Autodesk Inventor part; units mm, degrees
ref_plane "YZ Plane" through (0, 0, 0) normal (1, 0, 0) x (0, 1, 0)
ref_plane "XZ Plane" through (0, 0, 0) normal (0, 1, 0) x (-1, 0, 0)
ref_plane "XY Plane" through (0, 0, 0) normal (0, 0, 1) x (1, 0, 0)
sketch "Skizze1" plane through (0, 0, 0) normal (0, 0, 1) x (1, 0, 0)
  line L0 (-58, -45) -> (58, -45)
  line L1 (58, -45) -> (58, 45)
  line L2 (58, 45) -> (-58, 45)
  line L3 (-58, 45) -> (-58, -45)
  line L4 (-58, -45) -> (58, 45) construction
  line L5 (58, -45) -> (-58, 45) construction
  point P0 (0, 0)
  dimension "d0" = 116
  dimension "d1" = 90
extrude "Extrusion1" add sketch "Skizze1" along normal blind 15
sketch "Skizze2" plane through (0, 0, 15) normal (0, 0, 1) x (1, 0, 0)
  line L0 (58, -45) -> (58, 45)
  point P0 (0, 0)
  point P1 (47, 0)
  point P2 (58, 0)
  dimension "d11" = 11
hole "Bohrung1" at (47, 0, 15) direction (0, 0, -1) diameter 4.134 depth 13 tip angle 118
sketch "Skizze4" plane through (0, 0, 15) normal (0, 0, 1) x (1, 0, 0)
  line L0 (-58, -45) -> (58, -45)
  line L1 (58, -45) -> (58, 45)
  point P0 (0, 0)
  point P1 (-35.5, 16)
  point P2 (36, -10)
  dimension "d20" = 35
  dimension "d21" = 61
  dimension "d22" = 22
  dimension "d23" = 71.5
hole "Bohrung3" at (-35.5, 16, 15) at (36, -10, 15) direction (0, 0, -1) diameter 5.5 end through all counterbore diameter 10 counterbore depth 6.5
sketch "Skizze5" plane through (0, 0, 15) normal (0, 0, 1) x (1, 0, 0)
  line L0 (-58, 45) -> (-58, -45)
  circle A0 centre (47, 0) radius 2.067
  point P0 (0, 0)
  point P1 (-46.5721, 0)
  point P2 (-58, 0)
  dimension "d38" = 93.5721
hole "Bohrung4" at (-46.5721, 0, 15) direction (0, 0, -1) diameter 4.134 depth 13 tip angle 118
sketch "Skizze6" plane through (0, 0, 15) normal (0, 0, 1) x (1, 0, 0)
  circle A0 centre (-35.5, 16) radius 2.75
  point P0 (0, 0)
  point P1 (-35.5, -14)
  dimension "d39" = 30
hole "Bohrung5" at (-35.5, -14, 15) direction (0, 0, -1) diameter 5.5 depth 15 counterbore diameter 10 counterbore depth 6.5
sketch "Skizze7" plane through (0, 0, 15) normal (0, 0, 1) x (1, 0, 0)
  point P0 (0, 0)
  point P1 (-46.0168, 35.3976)
hole "Bohrung6" at (-46.0168, 35.3976, 15) direction (0, 0, -1) diameter 3 depth 8 tip angle 118
sketch "Skizze8" plane through (0, 0, 0) normal (0, 0, -1) x (-1, 0, 0)
  line L0 (58, -45) -> (-58, -45)
  line L1 (58, 45) -> (58, -45)
  point P0 (0, 0)
  point P1 (42.6552, 35)
  point P2 (24.6552, -15)
  point P3 (58, 0)
  dimension "d61" = 50
  dimension "d62" = 30
  dimension "d63" = 18
hole "Bohrung7" at (-42.6552, 35, 0) at (-24.6552, -15, 0) direction (0, 0, 1) diameter 4 depth 8 tip angle 118
sketch "Skizze10" plane through (0, 0, 0) normal (0, 0, -1) x (-1, 0, 0)
  line L0 (-58, -45) -> (-58, 45)
  line L1 (58, -45) -> (-58, -45)
  point P0 (0, 0)
  point P1 (-27, 1)
  point P2 (-45, -11)
  dimension "d71" = 18
  dimension "d72" = 31
  dimension "d73" = 34
  dimension "d74" = 12
hole "Bohrung8" at (27, 1, 0) at (45, -11, 0) direction (0, 0, 1) diameter 3 end through all
chamfer "Fasen1" distance 1 angle 45 12 edges at (58, 0, 0) (0, 45, 0) (-58, 0, 0) (0, -45, 0) (0, 45, 15) (-58, 45, 7.5) (58, 45, 7.5) (-58, 0, 15) (58, 0, 15) (-58, -45, 7.5) (58, -45, 7.5) (0, -45, 15)
properties part number "Grundplatte" material "Glas"
Model file for the job. Use its own axes, mm. A direction names the side the tool comes from. Round coordinates to 2 decimals unless told otherwise and drop trailing zeros. Loops run counter-clockwise (first coordinate to the right, second up) from the corner with the lowest first, then second, coordinate; pieces in that order, holes last.
1. Wall check: probe 1 along X at (y, z) = (1, 4.25); probe 2 along Y at (x, z) = (27, 12); probe 3 along Y at (x, z) = (-37, 1). Give the ranges that are in metal, low to high.
Check values:
probe 1: x = -58 to -48.38, -44.76 to 25.5, 28.5 to 45.19, 48.81 to 58
probe 2: y = -45 to -0.5, 2.5 to 45
probe 3: y = -45 to -16.3, -11.7 to 13.7, 18.3 to 45
2. Mould opens along Y. For faces 3 (the flat face through (1, 45, 7)), 4 (the conical face through (-42.994, 34.925, 8.993)), 5 (the flat face through (-58, 1, 7)) say: +Y half, -Y half, draft (parallel to the pull), parting line (faces both ways), or undercut.
Check values:
face 3: +Y half
face 4: undercut
face 5: draft
3. Tool access for faces 1 (the cylindrical face through (33.273, -9.642, 4.19)), 2 (the cylindrical face through (34.5, -14.77, 11.7)): list every direction of +Z, -Z, +X, -X, +Y, -Y with a clear straight run to the whole face (end or side of a thin tool).
Check values:
face 1: +Z, -Z
face 2: +Z
4. Drop a flat-ended pin along its axis: P1, Ø3, axis at x = -34.5, y = 14, coming from the +Z side. Give the stop position or say it passes through.
Check values:
P1: stops at z = 8.5
5. Band-saw the part on B-B, the plane z = 11. Count the separate pieces of the cut face and the enclosed holes in it, and give its area (3 significant figures).
Check values:
separate pieces: 1
enclosed holes: 8
area: 10,200 mm2
6. Band-saw the part on A-A, the plane x = -35.5. List the corners of the cut face in (y, z).
Check values:
outline: (-45, 1) - (-44, 0) - (-16.75, 0) - (-16.75, 8.5) - (-19, 8.5) - (-19, 15) - (-44, 15) - (-45, 14) - close; (-11.25, 0) - (13.25, 0) - (13.25, 8.5) - (11, 8.5) - (11, 15) - (-9, 15) - (-9, 8.5) - (-11.25, 8.5) - close; (18.75, 0) - (44, 0) - (45, 1) - (45, 14) - (44, 15) - (21, 15) - (21, 8.5) - (18.75, 8.5) - close
